Autodesk Inventor part; units mm, degrees
ref_plane "YZ Plane" through (0, 0, 0) normal (1, 0, 0) x (0, 1, 0)
ref_plane "XZ Plane" through (0, 0, 0) normal (0, 1, 0) x (-1, 0, 0)
ref_plane "XY Plane" through (0, 0, 0) normal (0, 0, 1) x (1, 0, 0)
sketch "Boceto1" plane through (0, 0, 0) normal (0, 0, 1) x (1, 0, 0)
  line L0 (-4.25, 9.25) -> (4.25, 9.25)
  line L1 (9.25, 4.25) -> (9.25, -4.25)
  line L2 (4.25, -9.25) -> (-4.25, -9.25)
  line L3 (-9.25, -4.25) -> (-9.25, 4.25)
  arc A0 (-4.25, 9.25) -> (-9.25, 4.25) centre (-4.25, 4.25) ccw
  arc A1 (-9.25, -4.25) -> (-4.25, -9.25) centre (-4.25, -4.25) ccw
  arc A2 (4.25, -9.25) -> (9.25, -4.25) centre (4.25, -4.25) ccw
  arc A3 (9.25, 4.25) -> (4.25, 9.25) centre (4.25, 4.25) ccw
extrude "Extrusión1" add sketch "Boceto1" against normal blind 2.5
sketch "Boceto3" plane through (0, 0, -2.5) normal (0, 0, -1) x (-1, 0, 0)
  line L0 (-5, -5) -> (5, -5)
  line L1 (5, -5) -> (5, 5)
  line L2 (5, 5) -> (-5, 5)
  line L3 (-5, 5) -> (-5, -5)
extrude "Extrusión2" add sketch "Boceto3" along normal blind 29
sketch "Boceto4" plane through (0, 0, 0) normal (0, 0, 1) x (1, 0, 0)
  line L0 (-3.65, 8.15) -> (3.65, 8.15)
  line L1 (8.15, 3.65) -> (8.15, -3.65)
  line L2 (3.65, -8.15) -> (-3.65, -8.15)
  line L3 (-8.15, -3.65) -> (-8.15, 3.65)
  arc A0 (3.65, -8.15) -> (8.15, -3.65) centre (3.65, -3.65) ccw
  arc A1 (-8.15, -3.65) -> (-3.65, -8.15) centre (-3.65, -3.65) ccw
  arc A2 (-3.65, 8.15) -> (-8.15, 3.65) centre (-3.65, 3.65) ccw
  arc A3 (8.15, 3.65) -> (3.65, 8.15) centre (3.65, 3.65) ccw
  line L4 (-2.5, 6) -> (2.5, 6)
  line L5 (6, 2.5) -> (6, -2.5)
  line L6 (2.5, -6) -> (-2.5, -6)
  line L7 (-6, -2.5) -> (-6, 2.5)
  arc A4 (6, 2.5) -> (2.5, 6) centre (2.5, 2.5) ccw
  arc A5 (2.5, -6) -> (6, -2.5) centre (2.5, -2.5) ccw
  arc A6 (-6, -2.5) -> (-2.5, -6) centre (-2.5, -2.5) ccw
  arc A7 (-2.5, 6) -> (-6, 2.5) centre (-2.5, 2.5) ccw
extrude "Extrusión3" add sketch "Boceto4" along normal blind 9.5
sketch "Boceto5" plane through (0, 0, -31.5) normal (0, 0, -1) x (-1, 0, 0)
  arc A0 (-1.4, 2.1909) -> (1.4, 2.1909) centre (0, 0) ccw
  line L0 (1.4, 2.1909) -> (-1.4, 2.1909)
  dimension "d36" = 5.2
  dimension "d37" = 2.8
extrude "Extrusión4" cut sketch "Boceto5" against normal blind 18
properties part number "_3DPrint"
The model under review builds one solid part; all positions refer to its coordinate system, in mm. A direction names the side the tool comes from. Give positions to 0.01 mm unless a question says otherwise; leave off trailing zeros. Loops run counter-clockwise (first coordinate to the right, second up) from the corner with the lowest first, then second, coordinate; pieces in that order, holes last. Notation, with made-up numbers: (-31.5, -1.5) -> (17.5, -1.5) arc R14 cw to (17.5, 19.5) -> close; hole circle Ø1 at (-11.5, 35). An arc over 180 degrees is marked (long way). Put each result on its own line as item: value. Start each with the question number.
1. We need section B-B on z = -25. State the section outline as (x, y) points, then the cut area to 3 significant figures.
2. For faces 1 (the face through (0, -8.15, 5)), 2 (the face through (6.867, -6.797, 4.684)), 3 (the face through (-5, 4.95, 4.68)), 4 (the face through (0, 2.191, -23)), list the 3-axis set-ups (+Z, -Z, +X, -X, +Y, -Y) from which the entire face can be reached by the end or side of a thin tool; tool diameter is ignored.
3. Mouldability with a two-part tool opening along X and no side actions: class faces 5 (the face through (7.75, -7.82, -1.23)), 6 (the face through (0.1, -2.6, -22.6)), 7 (the face through (0, -9.25, -1)) as released by +X, released by -X, zero draft, split by the parting line, or undercut.
4. We need section C-C on y = 0. State the section outline as (x, z) points, then the cut area to 4 significant figures.
5. We need section A-A on x = 0. State the section outline as (y, z) points, then the cut area to 3 significant figures.
6. Clearance check with flat-ended pins moving along their axes: P1, Ø4, axis at y = -2.5, z = -18, coming from the +X side; P2, Ø2.5, axis at y = -1, z = 7, coming from the +X side; P3, Ø1, axis at x = -2.5, y = -7, coming from the -Z side. State where each tip first meets the part, or that it passes through.
7. Wall thickness on probe 1 along X at (y, z) = (-1.75, 6.5); probe 2 along Z at (x, y) = (-6, -3.75); probe 3 along X at (y, z) = (-3.5, -5.5): over which ranges is each line inside the solid? List them lowest first.
8. We need section D-D on z = -10.5. State the section outline as (x, y) points.
Determined:
1. outline: (-5, -5) -> (5, -5) -> (5, 5) -> (-5, 5) -> close; hole (-1.4, 2.19) arc R2.6 ccw (long way) to (1.4, 2.19) -> close
1. area: 79.5 mm^2
2. face 1: +Z, +X, -X, -Y
2. face 2: +Z, +X, -Y
2. face 3: +Z
2. face 4: -Z
3. face 5: released by +X
3. face 6: undercut
3. face 7: zero draft
4. outline: (-9.25, -2.5) -> (-5, -2.5) -> (-5, -31.5) -> (-2.6, -31.5) -> (-2.6, -13.5) -> (2.6, -13.5) -> (2.6, -31.5) -> (5, -31.5) -> (5, -2.5) -> (9.25, -2.5) -> (9.25, 0) -> (8.15, 0) -> (8.15, 9.5) -> (6, 9.5) -> (6, 0) -> (-6, 0) -> (-6, 9.5) -> (-8.15, 9.5) -> (-8.15, 0) -> (-9.25, 0) -> close
4. area: 283.5 mm^2
5. outline: (-9.25, -2.5) -> (-5, -2.5) -> (-5, -31.5) -> (-2.6, -31.5) -> (-2.6, -13.5) -> (2.19, -13.5) -> (2.19, -31.5) -> (5, -31.5) -> (5, -2.5) -> (9.25, -2.5) -> (9.25, 0) -> (8.15, 0) -> (8.15, 9.5) -> (6, 9.5) -> (6, 0) -> (-6, 0) -> (-6, 9.5) -> (-8.15, 9.5) -> (-8.15, 0) -> (-9.25, 0) -> close
5. area: 291 mm^2
6. P1: x = 5
6. P2: x = 8.15
6. P3: z = -2.5
7. probe 1: -8.15 to -6, 6 to 8.15
7. probe 2: -2.5 to 9.5
7. probe 3: -5 to 5
8. outline: (-5, -5) -> (5, -5) -> (5, 5) -> (-5, 5) -> close
